from build123d import *

# Parameters (mm, degrees)
SKETCH_W     = 40
SKETCH_H     = 40
SKETCH_R     = 2.5
PAD_DEPTH    = 10
CHAMFER_SIZE = 1


with BuildPart() as part:
    # Sketch → Pad (new body)
    with BuildSketch(Plane.XY):
        Rectangle(SKETCH_W, SKETCH_H)
        with Locations((-10, 10)):
            Circle(SKETCH_R, mode=Mode.SUBTRACT)
    extrude(amount=PAD_DEPTH)

    # Sketch001 → Revolution (revolve)
    with BuildSketch(Plane(origin=(-10, 10, 0), x_dir=(1, 0, 0), z_dir=(0, -1, 0))):
        Polygon((2.5, 11.2), (3.3, 11.2), (4.5, 10), (2.5, 10), align=None)
    revolve(axis=Axis((-10, 10, 0), (0, 0, 1)))

    # Chamfer
    chamfer_edges = [part.edges().sort_by_distance(p)[0] for p in [
        (0, -20, 10),
        (-20, 0, 10),
        (0, 20, 10),
        (20, 0, 10),
    ]]
    chamfer(chamfer_edges, length=CHAMFER_SIZE)


solid = part.part
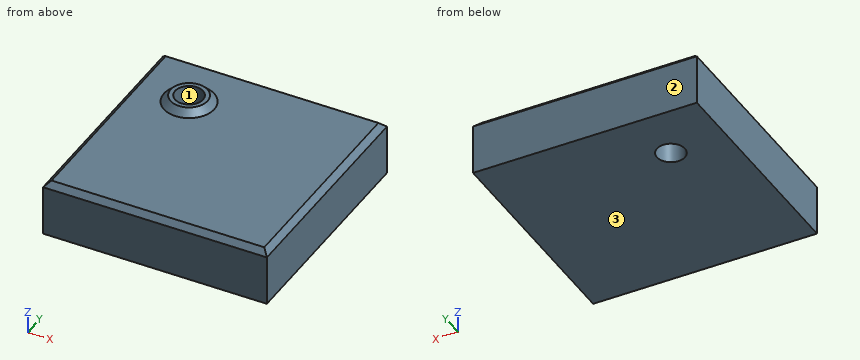
Work out the finished part from the listing and answer in its coordinate system (mm). Face numbers are marked on the shaded views. Coordinates: 2 decimals unless noted, no trailing zeros. Loops run counter-clockwise (first coordinate to the right, second up) from the corner with the lowest first, then second, coordinate; pieces in that order, holes last. Notation, with made-up numbers: (16, -30.5) -> (36, -30.5) arc R20 ccw to (36, -5.5) -> close; hole circle Ø1 at (-11.75, 59). An arc over 180 degrees is marked (long way). Write each question's results on one line, items separated by ' | '. Start each with the question number.
1) Consider line 1 along Y through (x, z) = (-10, 8.25); line 2 along Z through (x, y) = (-13, -16); line 3 along X through (y, z) = (11, 5.5). Determine where each line is inside the solid, lowest interval first.
2) Find section C-C on y = -2. Determine the outline of the cut face in (x, z).
3) The mould has two halves that part along Y. Classify the marked faces 1, 2 and 3: pulls with the +Y half, pulls with the -Y half, needs draft (parallel to the pull), parting line crosses it, or undercut.
4) Find section A-A on y = 10. Determine the outline of the cut face in (x, z), then the cut area to 3 significant figures.
5) Find section B-B on x = -10. Determine the outline of the cut face in (y, z).
Response values:
1) line 1: y = -20 to 7.5, 12.5 to 20 | line 2: z = 0 to 10 | line 3: x = -20 to -12.29, -7.71 to 20
2) outline: (-20, 0) -> (20, 0) -> (20, 9) -> (19, 10) -> (-19, 10) -> (-20, 9) -> close
3) face 1: undercut | face 2: pulls with the +Y half | face 3: needs draft
4) outline: (-20, 0) -> (-12.5, 0) -> (-12.5, 11.2) -> (-13.3, 11.2) -> (-14.5, 10) -> (-19, 10) -> (-20, 9) -> close; (-7.5, 0) -> (20, 0) -> (20, 9) -> (19, 10) -> (-5.5, 10) -> (-6.7, 11.2) -> (-7.5, 11.2) -> close | area: 352 mm^2
5) outline: (-20, 0) -> (7.5, 0) -> (7.5, 11.2) -> (6.7, 11.2) -> (5.5, 10) -> (-19, 10) -> (-20, 9) -> close; (12.5, 0) -> (20, 0) -> (20, 9) -> (19, 10) -> (14.5, 10) -> (13.3, 11.2) -> (12.5, 11.2) -> close
